Could you check a few things on this model? Use its own coordinates, in mm. Round coordinates to 2 decimals unless told otherwise and drop trailing zeros. Loops run counter-clockwise (first coordinate to the right, second up) from the corner with the lowest first, then second, coordinate; pieces in that order, holes last. Notation, with made-up numbers: (29, -15) -> (55, -15) arc R20 cw to (55, 22) -> close; hole circle Ø9 at (50.25, 22.5). An arc over 180 degrees is marked (long way). Put each result on its own line as item: value. Start each with the question number.
1. Imagine slicing it at C-C, the plane z = 0.4. Please give me the cut outline in (x, y).
2. I'm going to push a flat-ended pin straight in: P1, Ø3.5, axis at x = 0, y = -19.65, coming from the +Z side. Where does the tip first touch, or does it pass through?
3. I need wall thicknesses on line 1 (Y direction, x = 0, z = 1.2); line 2 (Y direction, x = -1.5, z = 0.1); line 3 (X direction, y = -6.5, z = 0.35). Which ranges of each line are inside material? Lowest first, please. Write a range as [from, to].
4. Imagine slicing it at B-B, the plane x = 0. Please give me the cut outline in (y, z), and give its area (3 significant figures).
Autodesk Inventor part; units mm, degrees
ref_plane "YZ Plane" through (0, 0, 0) normal (1, 0, 0) x (0, 1, 0)
ref_plane "XZ Plane" through (0, 0, 0) normal (0, 1, 0) x (-1, 0, 0)
ref_plane "XY Plane" through (0, 0, 0) normal (0, 0, 1) x (1, 0, 0)
sketch "Sketch1" plane through (0, 0, 0) normal (0, 0, 1) x (1, 0, 0)
  circle A0 centre (0, 19.65) radius 2.1828
  circle A1 centre (0, -19.65) radius 2.1828
  line L0 (-6.35, -26) -> (6.35, -26)
  line L1 (6.35, -26) -> (6.35, 26)
  line L2 (6.35, 26) -> (-6.35, 26)
  line L3 (-6.35, 26) -> (-6.35, -26)
  line L4 (-6.35, -26) -> (6.35, 26) construction
  line L5 (6.35, -26) -> (-6.35, 26) construction
  point P0 (0, 0)
  dimension "d0" = 4.3656
  dimension "d1" = 4.3656
  dimension "d2" = 19.65
  dimension "d3" = 39.3
  dimension "d4" = 19.65
  dimension "d5" = 12.7
  dimension "d6" = 6.35
extrude "Extrusion1" add sketch "Sketch1" along normal blind 1.5875
fillet "Fillet1" radius 0.7937 4 edges at (-6.35, 0, 0) (-6.35, 0, 1.5875) (6.35, 0, 0) (6.35, 0, 1.5875)
properties part number "Part C"
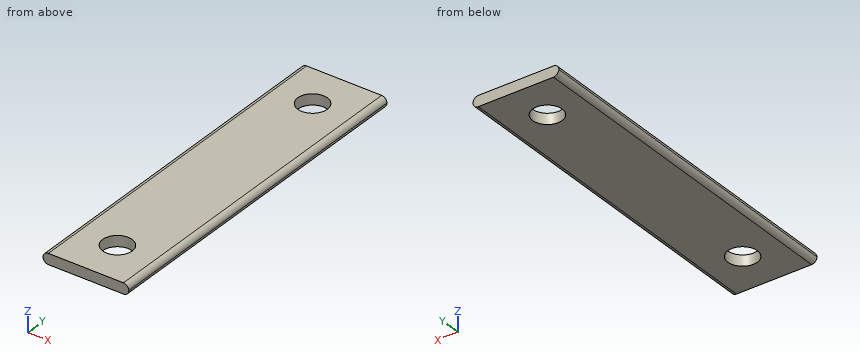
Entries:
1. outline: (-6.25, -26) -> (6.25, -26) -> (6.25, 26) -> (-6.25, 26) -> close; hole circle Ø4.37 at (0, -19.65); hole circle Ø4.37 at (0, 19.65)
2. P1: through
3. line 1: [-26, -21.83], [-17.47, 17.47], [21.83, 26]
3. line 2: [-26, -21.24], [-18.06, 18.06], [21.24, 26]
3. line 3: [-6.21, 6.21]
4. outline: (-26, 0) -> (-21.83, 0) -> (-21.83, 1.59) -> (-26, 1.59) -> close; (-17.47, 0) -> (17.47, 0) -> (17.47, 1.59) -> (-17.47, 1.59) -> close; (21.83, 0) -> (26, 0) -> (26, 1.59) -> (21.83, 1.59) -> close
4. area: 68.7 mm^2
